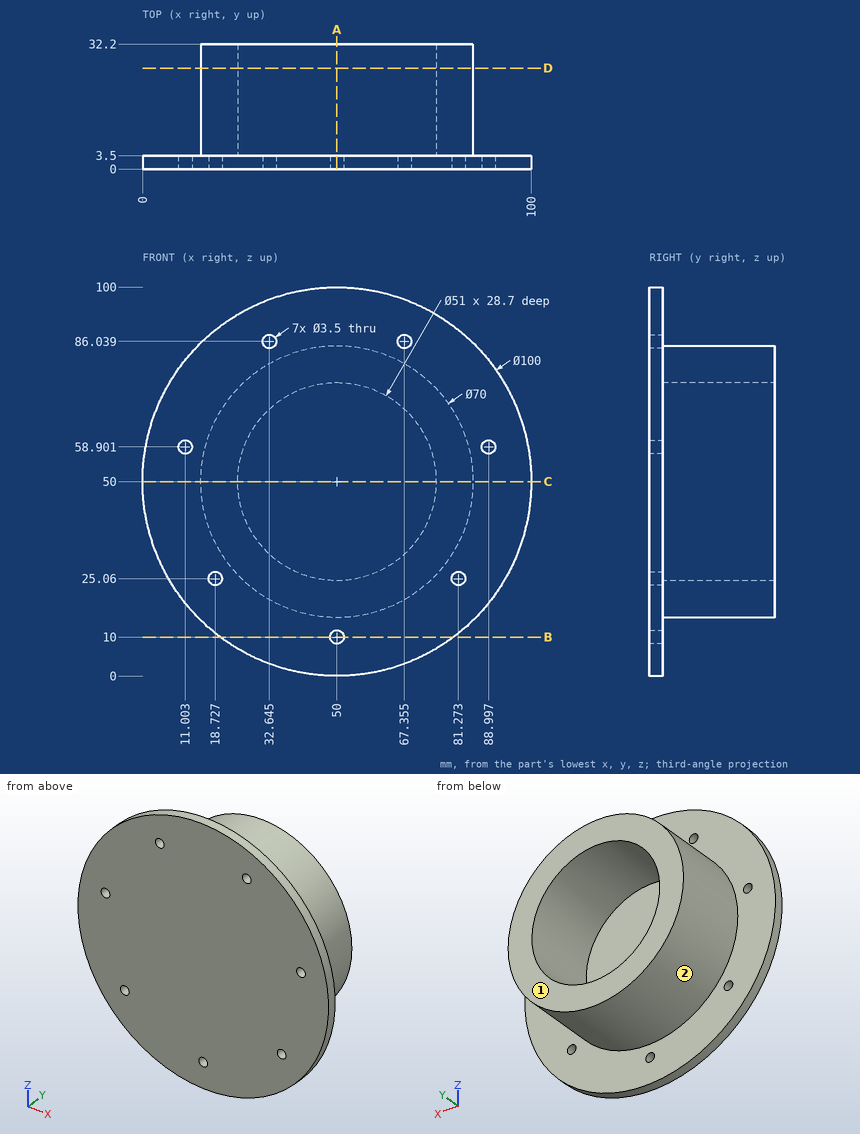
Geometry: see drawing. Coordinates: mm, zero at the bounding-box minimum. A direction names the side the tool comes from. Round coordinates to 2 decimals unless told otherwise and drop trailing zeros. Loops run counter-clockwise (first coordinate to the right, second up) from the corner with the lowest first, then second, coordinate; pieces in that order, holes last. Notation, with made-up numbers: (-19.5, -4) -> (30.5, -4) arc R13 cw to (30.5, 17) -> close; hole circle Ø4 at (44, 16.5). An arc over 180 degrees is marked (long way). Write each question's results on one line, items separated by ' | '.
1. Section C-C (z = 50). Return loops of the section in (x, y).
Geometry results:
outline: (0, 0) -> (100, 0) -> (100, 3.5) -> (85, 3.5) -> (85, 32.2) -> (75.5, 32.2) -> (75.5, 3.5) -> (24.5, 3.5) -> (24.5, 32.2) -> (15, 32.2) -> (15, 3.5) -> (0, 3.5) -> close
2. First-contact query: P1, Ø3, axis at x = 14.5, y = 4, coming from the -Z side; P2, Ø1, axis at x = 16, z = 76, coming from the +Y side; P3, Ø3, axis at y = 19.5, z = 76, coming from the +X side (1 decimal). Flat tips, straight axial feed; report the tip coordinate or a pass-through.
Geometry results:
P1: z = 13.42 | P2: y = 3.5 | P3: x = 75
3. Section A-A (x = 50). Return loops of the section in (y, z), and give its area (3 significant figures).
Geometry results:
outline: (0, 0) -> (3.5, 0) -> (3.5, 8.25) -> (0, 8.25) -> close; (0, 11.75) -> (3.5, 11.75) -> (3.5, 15) -> (32.2, 15) -> (32.2, 24.5) -> (3.5, 24.5) -> (3.5, 75.5) -> (32.2, 75.5) -> (32.2, 85) -> (3.5, 85) -> (3.5, 100) -> (0, 100) -> close | area: 883 mm2
4. Ray query, line 1 (Y direction, x = 48.5, z = 91); line 2 (Z direction, x = 49.5, y = 26) (1 decimal); line 3 (Z direction, x = 34.5, y = 12). Return the intervals inside material, ascending. Write a range as from..to.
Geometry results:
line 1: 0..3.5 | line 2: 15..24.5, 75.5..85 | line 3: 18.62..29.75, 70.25..81.38
5. Section D-D (y = 26). Return loops of the section in (x, z), and give its area (3 significant figures).
Geometry results:
outline: circle Ø70 at (50, 50); hole circle Ø51 at (50, 50) | area: 1,810 mm2
6. Set-up query: the marked faces 1 and 2. Return all of +Z, -Z, +X, -X, +Y, -Y with unobstructed straight access to the full face (end or side cutting, diameter ignored); none if empty.
Geometry results:
face 1: +Z, -Z, +X, -X, +Y | face 2: +Y
7. Section B-B (z = 10). Return loops of the section in (x, y), and give its area (3 significant figures).
Geometry results:
outline: (20, 0) -> (48.25, 0) -> (48.25, 3.5) -> (20, 3.5) -> close; (51.75, 0) -> (80, 0) -> (80, 3.5) -> (51.75, 3.5) -> close | area: 198 mm2
